Build history of the part. All positions in model axes, mm. A direction names the side the tool comes from. Round coordinates to 2 decimals unless told otherwise and drop trailing zeros. Loops run counter-clockwise (first coordinate to the right, second up) from the corner with the lowest first, then second, coordinate; pieces in that order, holes last. Notation, with made-up numbers: M 25.25,47.5 L 37.25,47.5 A17 cw 37.25,72.5 Z; hole C 44.25,53 d2. An arc over 180 degrees is marked long. One line per item, written item: value.
```python
from build123d import *

# Parameters (mm, degrees)
SKETCH_1_R          = 2.5
EXTRUDE_1_DEPTH     = 6
SKETCH_2_R          = 2.5
SKETCH_3_R          = 1.5
SKETCH_5_R          = 1.5
SKETCH_6_R          = 1.15
SKETCH_7_R          = 1
CUT_EXTRUDE_1_DEPTH = 8.5
SKETCH_8_R          = 1.25
CUT_EXTRUDE_2_DEPTH = 8.5
CHAMFER_1_SIZE      = 0.5
FILLET_1_R          = 0.1


with BuildPart() as part:
    # 草图1 → 凸台-拉伸1 (new body)
    with BuildSketch(Plane(origin=(0, 0, 0), x_dir=(1, 0, 0), z_dir=(0, 1, 0))):
        with Locations(Location((0, 0, 0), (0, 0, 270))):
            Circle(SKETCH_1_R)
    extrude(amount=EXTRUDE_1_DEPTH)

    # 草图2 → 放样1 section 0
    with BuildSketch(Plane(origin=(0, 6, 0), x_dir=(1, 0, 0), z_dir=(0, 1, 0))):
        Circle(SKETCH_2_R)
    # 草图3 → 放样1 section 1
    with BuildSketch(Plane(origin=(0, 7, 0), x_dir=(1, 0, 0), z_dir=(0, 1, 0))):
        Circle(SKETCH_3_R)
    loft()

    # 草图4 → 旋转1 (revolve)
    with BuildSketch(Plane.XY, mode=Mode.PRIVATE) as revolve_1_sk:
        with BuildLine():
            Line((0, 7), (0, 8.5))
            Line((0, 8.5), (0, 10))
            ThreePointArc((0, 10), (-1.060660172, 9.560660172), (-1.5, 8.5))
            Line((-1.5, 8.5), (-1.5, 7))
            Line((-1.5, 7), (0, 7))
        make_face()
    revolve(revolve_1_sk.sketch.rotate(Axis((0, 8.5, 0), (0, 1, 0)), 270), axis=Axis((0, 8.5, 0), (0, 1, 0)))

    # 草图5 → 放样2 section 0
    with BuildSketch(Plane.XY):
        with Locations((0, 8.5)):
            Circle(SKETCH_5_R)
    # 草图6 → 放样2 section 1
    with BuildSketch(Plane.XY.offset(8.5)):
        with Locations((0, 8.5)):
            Circle(SKETCH_6_R)
    loft()

    # 草图7 → 切除-拉伸1 (cut)
    with BuildSketch(Plane.XY.offset(8.5)):
        with Locations((0, 8.5)):
            Circle(SKETCH_7_R)
    extrude(amount=-CUT_EXTRUDE_1_DEPTH, mode=Mode.SUBTRACT)

    # 草图8 → 切除-拉伸2 (cut)
    with BuildSketch(Plane.XZ):
        with Locations(Location((0, 0, 0), (0, 0, 270))):
            Circle(SKETCH_8_R)
    extrude(amount=-CUT_EXTRUDE_2_DEPTH, mode=Mode.SUBTRACT)

    # 倒角1
    chamfer_1_edges = [part.edges().sort_by_distance(p)[0] for p in [
        (0, 0, -2.5),
        (0, 0, 1.25),
    ]]
    chamfer(chamfer_1_edges, length=CHAMFER_1_SIZE)

    # 圆角1
    fillet_1_edges = [part.edges().sort_by_distance(p)[0] for p in [
        (-1.15, 8.5, 8.5),
    ]]
    fillet(fillet_1_edges, radius=FILLET_1_R)


solid = part.part
```
Item 1: Drop flat-ended pins along their axis: P1, Ø1.5, axis at x = 0.5, z = 0.5, coming from the +Y side; P2, Ø1.5, axis at x = -1.5, z = 5, coming from the -Y side; P3, Ø1.2, axis at x = 0, y = 8.5, coming from the +Z side; P4, Ø2, axis at x = 0.5, z = 0, coming from the -Y side. Give the stop position or say it passes through.
Check values:
P1: stops at y = 10
P2: stops at y = 7.44
P3: stops at z = 0
P4: stops at y = 0.25
Item 2: Slice it at A-A, the plane y = 5. Give the cut face in (x, z).
Check values:
outline: C 0,0 d5; hole C 0,0 d2.5
Item 3: Wall check: line 1 along Z through (x, y) = (-0.1, 5); line 2 along Y through (x, z) = (0, 4). Give the ranges that are in metal, low to high.
Check values:
line 1: z = -2.5 to -1.25, 1.25 to 2.5
line 2: y = 7.16 to 7.5, 9.5 to 9.84
Item 4: Which spindle directions (+Z, -Z, +X, -X, +Y, -Y) get a long thin tool onto all of the face, cutting with end or side? Do faces 1 (the face through (-0.13, 9.49, 4.31)), 2 (the face through (0.38, 4.44, -1.19)). Say none if no direction does.
Check values:
face 1: +Z
face 2: -Y
Item 5: Pull direction Y, two halves, no side cores. Call faces 3 (the face through (-0.45, 7.74, -1.43)), 4 (the face through (0, 9, 0)), 5 (the face through (0, 8.5, -0.5)): pulls with the +Y half, pulls with the -Y half, needs draft (parallel to the pull), parting line crosses it, or undercut.
Check values:
face 3: undercut
face 4: needs draft
face 5: pulls with the -Y half
Item 6: Slice it at B-B, the plane z = 6.75. Give the cut face in (x, y), and give its area (3 significant figures).
Check values:
outline: C 0,8.5 d2.44; hole C 0,8.5 d2
area: 1.55 mm2
